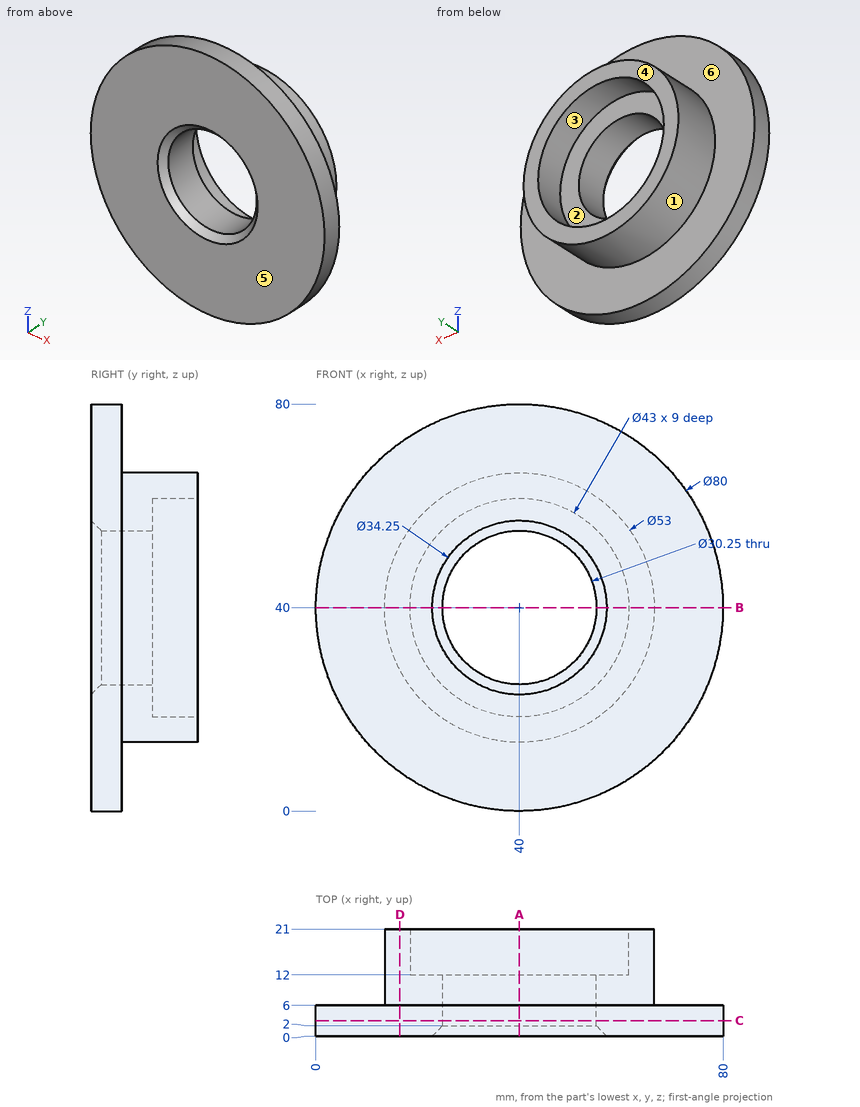
Study the drawing (mm; zero at the part's minimum x, y, z) and answer. A direction names the side the tool comes from. Coordinates: 2 decimals unless noted, no trailing zeros. Loops run counter-clockwise (first coordinate to the right, second up) from the corner with the lowest first, then second, coordinate; pieces in that order, holes last. Notation, with made-up numbers: M 76.25,29.25 L 105.25,29.25 A9 ccw 105.25,37.25 Z; hole C 61,16 d1. An arc over 180 degrees is marked long. Answer as a JSON object with one key per item and string values. Group by question number.
Item 1: Consider L1, parallel to Z at x = 40, y = 17.25; L2, parallel to Y at x = 30, z = 75; L3, parallel to Y at x = 54.5, z = 52. Determine where each line is inside the solid, lowest interval first.
Item 2: Section B-B (z = 40) is taken. Write down the section's boundary in (x, y) (3 decimals).
Item 3: Section A-A (x = 40) is taken. Write down the section's boundary in (y, z) (3 decimals).
Item 4: Determine the mould class of the marked faces 1, 2, 3 and 4 for opening direction X: +X half, -X half, draft (parallel to the pull), parting line (faces both ways), or undercut.
Item 5: Section C-C (y = 3) is taken. Write down the section's boundary in (x, z) (3 decimals), and give its area (3 significant figures).
Item 6: Section D-D (x = 16.5) is taken. Write down the section's boundary in (y, z), and give its area (3 significant figures).
Item 7: Which of the six approach directions +Z, -Z, +X, -X, +Y, -Y give full straight-line access (tool end or side, diameter ignored) to the marked faces 5 and 6?
Item 8: Each of these flat-tipped pins is pushed along its axis until it touches: P1, Ø10, axis at y = 8.5, z = 35.5, coming from the -X side; P2, Ø3, axis at y = 15.5, z = 28, coming from the +X side; P3, Ø6, axis at x = 17, y = 4.5, coming from the -Z side. Where does it stop, or does it pass through?
Solved:
{
 "1": {"L1": "z = 13.5 to 18.5, 61.5 to 66.5", "L2": "y = 0 to 6", "L3": "y = 0 to 12"},
 "2": {"outline": "M 0,0 L 22.875,0 L 24.875,2 L 24.875,12 L 18.5,12 L 18.5,21 L 13.5,21 L 13.5,6 L 0,6 Z; M 55.125,2 L 57.125,0 L 80,0 L 80,6 L 66.5,6 L 66.5,21 L 61.5,21 L 61.5,12 L 55.125,12 Z"},
 "3": {"outline": "M 0,0 L 6,0 L 6,13.5 L 21,13.5 L 21,18.5 L 12,18.5 L 12,24.875 L 2,24.875 L 0,22.875 Z; M 0,57.125 L 2,55.125 L 12,55.125 L 12,61.5 L 21,61.5 L 21,66.5 L 6,66.5 L 6,80 L 0,80 Z"},
 "4": {"face 1": "parting line", "face 2": "undercut", "face 3": "undercut", "face 4": "draft"},
 "5": {"outline": "C 40,40 d80; hole C 40,40 d30.25", "area": "4,310 mm2"},
 "6": {"outline": "M 0,7.63 L 6,7.63 L 6,27.75 L 21,27.75 L 21,52.25 L 6,52.25 L 6,72.37 L 0,72.37 Z", "area": "756 mm2"},
 "7": {"face 5": "+Z, -Z, +X, -X, -Y", "face 6": "+Y"},
 "8": {"P1": "stops at x = 0", "P2": "stops at x = 64.33", "P3": "stops at z = 5.36"}
}
